Geometry check sheet. Reference: the model listing, model coordinates, mm. A direction names the side the tool comes from. Coordinates: 2 decimals unless noted, no trailing zeros. Order: outer loops, then holes, each group sorted by start corner. A loop starts at its lowest first (then second) coordinate and runs counter-clockwise, first axis right, second up. Notation, with made-up numbers: (-24.75, 69) - (-4.75, 69) arc R31 cw to (-4.75, 102) - close; hole circle Ø9 at (-6.75, 26). An arc over 180 degrees is marked (long way). Use CSV: the item, a comma, the result in double quotes. Start each with the question number.
1) Thickness scan on probe 1 along Y at (x, z) = (-5.5, 18); probe 2 along X at (y, z) = (-3.5, 25.5); probe 3 along Z at (x, y) = (-8, 19). Record the ranges inside material, lowest first. Write a range as [from, to].
2) Sectioned sample at B-B, the plane x = 23. Record the cut outline in (y, z), and give its area (3 significant figures).
3) Sectioned sample at A-A, the plane z = 28. Record the cut outline in (x, y).
4) Depth check by flat-ended pin: P1, Ø3, axis at x = 38, z = 34, coming from the +Y side; P2, Ø3, axis at y = 4, z = 19.5, coming from the -X side; P3, Ø5, axis at x = -4, z = 16.5, coming from the +Y side; P4, Ø1, axis at x = -33.5, z = 25, coming from the -Y side. Enter the tip coordinate at first touch or a pass-through.
5) Tool access check on faces 5 (the flat face through (-27.518, 1, 28)), 6 (the cylindrical face through (46, -17.1, 12.5)), 7 (the cylindrical face through (-41.01, 20.03, 12.51)), 8 (the cylindrical face through (-33.12, 1.52, 15.57)), 9 (the cylindrical face through (48.084, 1.244, 10.57)). Record the directions out of +Z, -Z, +X, -X, +Y, -Y that give a thin tool (end or side, any length) a straight path to the whole face; none if there is none.
6) Sectioned sample at C-C, the plane y = 2.5. Record the cut outline in (x, z), and give its area (3 significant figures).
7) Draft check along X on faces 1 (the cylindrical face through (46.91, 1.24, 14.4)), 2 (the cylindrical face through (2.06, -9.15, 15.57)), 3 (the cylindrical face through (-31.014, -7.12, 28.661)), 4 (the flat face through (2, 2, 15)). Enter one of: released by +X, released by -X, zero draft, split by the parting line, or undercut.
from build123d import *

# Parameters (mm, degrees)
F0_W     = 100
F0_H     = 50
F1_DEPTH = 10
F2_W     = 90
F2_H     = 40
F3_DEPTH = 5
F4_W     = 70
F4_H     = 20
F5_DEPTH = 25
F6_W     = 60
F6_H     = 10
F7_DEPTH = 25
F8_R     = 5
F9_R     = 5
F10_R    = 5
F11_R    = 2


with BuildPart() as f1:
    # F0 (on Top) → F1 (new body)
    with BuildSketch(Plane.XY):
        with Locations((2.482289, 1.45373)):
            Rectangle(F0_W, F0_H)
    extrude(amount=F1_DEPTH)

    # F2 (on face) → F3 (join)
    with BuildSketch(Plane.XY.offset(10)):
        with Locations((2.482289, 1.45373)):
            Rectangle(F2_W, F2_H)
    extrude(amount=F3_DEPTH)

    # F4 (on face) → F5 (join)
    with BuildSketch(Plane.XY.offset(15)):
        with Locations((2.482289, 1.45373)):
            Rectangle(F4_W, F4_H)
    extrude(amount=F5_DEPTH)

    # F6 (on face) → F7 (cut)
    with BuildSketch(Plane.XY.offset(40)):
        with Locations((2.482289, 1.45373)):
            Rectangle(F6_W, F6_H)
    extrude(amount=-F7_DEPTH, mode=Mode.SUBTRACT)

    # F8
    f8_edges = [f1.edges().sort_by_distance(p)[0] for p in [
        (37.482289, -8.54627, 27.5),
        (37.482289, 11.45373, 27.5),
        (-32.517711, -8.54627, 27.5),
        (-32.517711, 11.45373, 27.5),
    ]]
    fillet(f8_edges, radius=F8_R)

    # F9
    f9_edges = [f1.edges().sort_by_distance(p)[0] for p in [
        (52.482289, 26.45373, 5),
        (-47.517711, -23.54627, 5),
        (-47.517711, 26.45373, 5),
        (52.482289, -23.54627, 5),
    ]]
    fillet(f9_edges, radius=F9_R)

    # F10
    f10_edges = [f1.edges().sort_by_distance(p)[0] for p in [
        (47.482289, -18.54627, 12.5),
        (-42.517711, -18.54627, 12.5),
        (47.482289, 21.45373, 12.5),
        (-42.517711, 21.45373, 12.5),
    ]]
    fillet(f10_edges, radius=F10_R)

    # F11
    f11_edges = [f1.edges().sort_by_distance(p)[0] for p in [
        (2.482289, 11.45373, 15),
        (2.482289, 21.45373, 15),
        (2.482289, 21.45373, 10),
        (2.482289, 26.45373, 10),
    ]]
    fillet(f11_edges, radius=F11_R)


solid = f1.part
Evaluation:
1,probe 1,"[-8.55, -3.55], [6.45, 11.45]"
1,probe 2,"[-32.52, -27.52], [32.48, 37.48]"
1,probe 3,"[0, 15]"
2,outline,"(-23.55, 0) - (26.45, 0) - (26.45, 8) arc R2 ccw to (24.45, 10) - (23.45, 10) arc R2 cw to (21.45, 12) - (21.45, 13) arc R2 ccw to (19.45, 15) - (13.45, 15) arc R2 cw to (11.45, 17) - (11.45, 40) - (6.45, 40) - (6.45, 15) - (-3.55, 15) - (-3.55, 40) - (-8.55, 40) - (-8.55, 17) arc R2 cw to (-10.55, 15) - (-16.55, 15) arc R2 ccw to (-18.55, 13) - (-18.55, 12) arc R2 cw to (-20.55, 10) - (-21.55, 10) arc R2 ccw to (-23.55, 8) - close"
2,area,"950 mm²"
3,outline,"(-32.52, -3.55) arc R5 ccw to (-27.52, -8.55) - (32.48, -8.55) arc R5 ccw to (37.48, -3.55) - (37.48, 6.45) arc R5 ccw to (32.48, 11.45) - (-27.52, 11.45) arc R5 ccw to (-32.52, 6.45) - close; hole (-27.52, -3.55) - (32.48, -3.55) - (32.48, 6.45) - (-27.52, 6.45) - close"
4,P1,"y = 9.43"
4,P2,"x = -32.52"
4,P3,"y = 21.19"
4,P4,"through"
5,face 5,"+Z"
5,face 6,"+Z, +X, -Y"
5,face 7,"+Z, -X, +Y"
5,face 8,"+Z, -X, +Y, -Y"
5,face 9,"+Z, +X, +Y, -Y"
6,outline,"(-47.52, 0) - (52.48, 0) - (52.48, 8) arc R2 ccw to (50.48, 10) - (49.48, 10) arc R2 cw to (47.48, 12) - (47.48, 13) arc R2 ccw to (45.48, 15) - (39.48, 15) arc R2 cw to (37.48, 17) - (37.48, 40) - (32.48, 40) - (32.48, 15) - (-27.52, 15) - (-27.52, 40) - (-32.52, 40) - (-32.52, 17) arc R2 cw to (-34.52, 15) - (-40.52, 15) arc R2 ccw to (-42.52, 13) - (-42.52, 12) arc R2 cw to (-44.52, 10) - (-45.52, 10) arc R2 ccw to (-47.52, 8) - close"
6,area,"1,700 mm²"
7,face 1,"released by +X"
7,face 2,"zero draft"
7,face 3,"released by -X"
7,face 4,"undercut"
